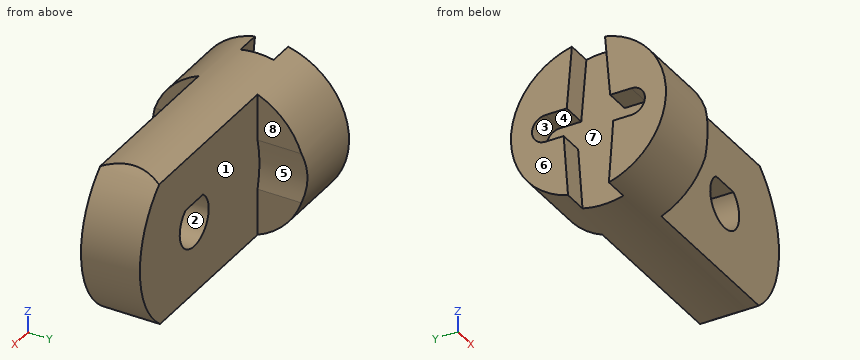
```python
from build123d import *

# Parameters (mm, degrees)
SKETCH_1_W                = 50
SKETCH_1_H                = 40
EXTRUDE_1_DEPTH           = 8
CHAMFER_1_SIZE            = 10
SKETCH_2_R                = 1.55
CUT_EXTRUDE_1_DEPTH       = 10
EXTRUDE_2_DEPTH           = 50
EXTRUDE_2_DEPTH_BACK      = 15
SKETCH_3_R                = 12.5
SKETCH_4_R                = 1.7
CUT_EXTRUDE_2_DEPTH       = 15
CUT_EXTRUDE_START         = -20
CUT_EXTRUDE_3_DEPTH       = 20
SKETCH_7_R                = 16.5
CUT_EXTRUDE_8_DEPTH       = 33
CUT_EXTRUDE_9_DEPTH       = 20
CHAMFER_3_SIZE            = 2
SKETCH_10_OUTSIDE_W       = 49.114
SKETCH_10_OUTSIDE_H       = 64.114
SKETCH_10_OUTSIDE_R       = 12.5
CUT_EXTRUDE_10_DEPTH      = 10
CHAMFER_4_SIZE            = 10
SKETCH_12_W               = 1.5
SKETCH_12_H               = 20
SKETCH_14_W               = 12
SKETCH_14_H               = 23
CUT_EXTRUDE_11_DEPTH      = 3
CUT_EXTRUDE_12_DEPTH      = 4.2
SKETCH_16_R               = 1.1
CUT_EXTRUDE_13_DEPTH      = 5
SKETCH_17_R               = 3.372674955
EXTRUDE_3_DEPTH           = 4
SKETCH_18_R               = 1.1
CUT_EXTRUDE_14_DEPTH      = 4
SKETCH_20_R               = 4
CUT_EXTRUDE_15_DEPTH      = 4
CUT_EXTRUDE_16_DEPTH      = 80.355214185
CUT_EXTRUDE_16_DEPTH_BACK = 80.355214185
SKETCH_21_W               = 47.755098741
SKETCH_21_H               = 76.122443719
SKETCH_26_R               = 4
CUT_EXTRUDE_19_DEPTH      = 20
SKETCH_28_W               = 34.99561618
SKETCH_28_H               = 41.128829021
CUT_EXTRUDE_20_DEPTH      = 10
SKETCH_29_W               = 7.599941767
SKETCH_29_H               = 6.479768366
EXTRUDE_6_DEPTH           = 9.5
SKETCH_24_R               = 12.607397707
CUT_EXTRUDE_21_DEPTH      = 15
CUT_EXTRUDE_22_DEPTH      = 4


# Read off the part's stored shape, not the designer's step: 切除-拉伸3
with BuildPart() as part:
    # 草图1 → 凸台-拉伸1 (new body)
    with BuildSketch(Plane.XY):
        Rectangle(SKETCH_1_W, SKETCH_1_H)
    extrude(amount=EXTRUDE_1_DEPTH)

    # 倒角1
    chamfer_1_edges = [part.edges().sort_by_distance(p)[0] for p in [
        (-25, -20, 4),
        (-25, 20, 4),
    ]]
    chamfer(chamfer_1_edges, length=CHAMFER_1_SIZE)

    # 草图2 → 切除-拉伸1 (cut)
    with BuildSketch(Plane.XY.offset(8)):
        with Locations((-2, -10)):
            Circle(SKETCH_2_R)
        with Locations((-2, 10)):
            Circle(SKETCH_2_R)
    extrude(amount=-CUT_EXTRUDE_1_DEPTH, mode=Mode.SUBTRACT)

    # 草图3 → 凸台-拉伸2 (add, two sides: drawn at the far end of the back side and taken through both)
    with BuildSketch(Plane(origin=(25, 0, 0), x_dir=(0, 0, -1), z_dir=(1, 0, 0)).offset(-EXTRUDE_2_DEPTH_BACK)):
        with Locations(Location((-4, 0, 0), (0, 0, 251.337075115))):
            Circle(SKETCH_3_R)
    extrude(amount=EXTRUDE_2_DEPTH + EXTRUDE_2_DEPTH_BACK)

    # 草图4 → 切除-拉伸2 (cut)
    with BuildSketch(Plane.XY.offset(8)):
        with Locations((-19.690178066, -4)):
            Circle(SKETCH_4_R)
        with Locations((-19.690178066, 4)):
            Circle(SKETCH_4_R)
    extrude(amount=-CUT_EXTRUDE_2_DEPTH, mode=Mode.SUBTRACT)

    # 切除-拉伸3 outline → 切除-拉伸3 (cut)
    with BuildSketch(Plane(origin=(75, 0, 0), x_dir=(0, 0, -1), z_dir=(1, 0, 0)).offset(CUT_EXTRUDE_START)):
        with BuildLine():
            Line((7.56233108, -4.75), (-15.56233108, -4.75))
            ThreePointArc((-15.56233108, -4.75), (-4, -12.5), (7.56233108, -4.75))
        make_face()
        with BuildLine():
            ThreePointArc((7.56233108, 4.75), (-4, 12.5), (-15.56233108, 4.75))
            Line((-15.56233108, 4.75), (7.56233108, 4.75))
        make_face()
    extrude(amount=CUT_EXTRUDE_3_DEPTH, mode=Mode.SUBTRACT)

    # 草图7 → 切除-拉伸8 (cut)
    with BuildSketch(Plane.XZ.offset(4.75)):
        with Locations((58.5, 4)):
            Circle(SKETCH_7_R)
    cut_extrude_8 = extrude(amount=CUT_EXTRUDE_8_DEPTH, mode=Mode.SUBTRACT)

    # 镜向1: 切除-拉伸8 across plane
    add(cut_extrude_8.mirror(Plane.ZX), mode=Mode.SUBTRACT)

    # 草图8 → 切除-拉伸9 (cut)
    with BuildSketch(Plane.XZ.offset(4.75)):
        with BuildLine():
            Line((60, 19.107397707), (75.764252489, 33.62580965))
            Line((75.764252489, 33.62580965), (78.826270749, -18.347337912))
            Line((78.826270749, -18.347337912), (60, -10.892602293))
            ThreePointArc((60, -10.892602293), (75, 4.107397707), (60, 19.107397707))
        make_face()
    extrude(amount=-CUT_EXTRUDE_9_DEPTH, mode=Mode.SUBTRACT)

    # 倒角3
    chamfer_3_edges = [part.edges().sort_by_distance(p)[0] for p in [
        (10, 0, 16.5),
        (10, 0, -8.5),
    ]]
    chamfer(chamfer_3_edges, length=CHAMFER_3_SIZE)

    # 草图10 outside → 切除-拉伸10 (cut)
    with BuildSketch(Plane(origin=(25, 0, 0), x_dir=(0, 0, -1), z_dir=(1, 0, 0))):
        with Locations((-4, 0)):
            Rectangle(SKETCH_10_OUTSIDE_W, SKETCH_10_OUTSIDE_H)
        with Locations((-4.107397707, 0)):
            Circle(SKETCH_10_OUTSIDE_R, mode=Mode.SUBTRACT)
    extrude(amount=-CUT_EXTRUDE_10_DEPTH, mode=Mode.SUBTRACT)

    # 倒角4
    # the kernel refuses this chamfer: 10 mm, written as the material it takes off along each edge
    with BuildSketch(Plane(origin=(15, -20, -25.71682988), x_dir=(-0.9996219169112968, -0.027495876610586317, 0), z_dir=(0, 0, 1))) as chamfer_4_piece_1_section:
        Polygon((CHAMFER_4_SIZE * 0.999621916911, -CHAMFER_4_SIZE * 0.0274958766106), (-CHAMFER_4_SIZE * 0.0274958766106, -CHAMFER_4_SIZE * 0.999621916911), (0, 0), align=None)
    chamfer_4_piece_1 = extrude(amount=59.433659759, mode=Mode.PRIVATE)
    chamfer_4_piece_1 = chamfer_4_piece_1 - Plane(origin=(11.669205873, 0, 4.107397707), x_dir=(0, 0, -1), z_dir=(1, 0, 0)) * Cylinder(12.5, 159, mode=Mode.PRIVATE)
    add(chamfer_4_piece_1, mode=Mode.SUBTRACT)
    with BuildSketch(Plane(origin=(15, 20, 33.71682988), x_dir=(-0.9996219169112968, 0.027495876610586317, 0), z_dir=(0, 0, -1))) as chamfer_4_piece_2_section:
        Polygon((CHAMFER_4_SIZE * 0.999621916911, -CHAMFER_4_SIZE * 0.0274958766106), (-CHAMFER_4_SIZE * 0.0274958766106, -CHAMFER_4_SIZE * 0.999621916911), (0, 0), align=None)
    chamfer_4_piece_2 = extrude(amount=59.433659759, mode=Mode.PRIVATE)
    chamfer_4_piece_2 = chamfer_4_piece_2 - Plane(origin=(11.669205873, 0, 4.107397707), x_dir=(0, 0, -1), z_dir=(1, 0, 0)) * Cylinder(12.5, 159, mode=Mode.PRIVATE)
    add(chamfer_4_piece_2, mode=Mode.SUBTRACT)

    # 草图12 → 切除-旋转2 (revolve, cut)
    with BuildSketch(Plane(origin=(0, 0, 0), x_dir=(1, 0, 0), z_dir=(0, 1, 0))):
        with Locations((14.75, 8.392602293)):
            Rectangle(SKETCH_12_W, SKETCH_12_H)
    revolve(axis=Axis((50, 0, 4.107397707), (-1, 0, 0)), mode=Mode.SUBTRACT)

    # 草图14 → 切除-拉伸11 (cut)
    with BuildSketch(Plane(origin=(0, 0, 0), x_dir=(-1, 0, 0), z_dir=(0, 0, -1))):
        with Locations((2, 4.65)):
            Rectangle(SKETCH_14_W, SKETCH_14_H)
    extrude(amount=-CUT_EXTRUDE_11_DEPTH, mode=Mode.SUBTRACT)

    # 草图15 → 切除-拉伸12 (cut)
    with BuildSketch(Plane(origin=(0, 0, 3), x_dir=(-1, 0, 0), z_dir=(0, 0, -1))):
        with BuildLine():
            ThreePointArc((4.631967524, 4.49702381), (2, 16.1), (-0.631967524, 4.49702381))
            ThreePointArc((-0.631967524, 4.49702381), (2, 0.95), (4.631967524, 4.49702381))
        make_face()
    extrude(amount=-CUT_EXTRUDE_12_DEPTH, mode=Mode.SUBTRACT)

    # 草图16 → 切除-拉伸13 (cut)
    with BuildSketch(Plane(origin=(0, 0, 0), x_dir=(-1, 0, 0), z_dir=(0, 0, -1))):
        with Locations((2, 18.3)):
            Circle(SKETCH_16_R)
    extrude(amount=-CUT_EXTRUDE_13_DEPTH, mode=Mode.SUBTRACT)

    # 草图17 → 凸台-拉伸3 (add)
    with BuildSketch(Plane(origin=(0, 0, 0), x_dir=(-1, 0, 0), z_dir=(0, 0, -1))):
        with Locations((2, -10)):
            Circle(SKETCH_17_R)
    extrude(amount=-EXTRUDE_3_DEPTH)

    # 草图18 → 切除-拉伸14 (cut)
    with BuildSketch(Plane(origin=(0, 0, 0), x_dir=(-1, 0, 0), z_dir=(0, 0, -1))):
        with Locations((2, -9)):
            Circle(SKETCH_18_R)
    extrude(amount=-CUT_EXTRUDE_14_DEPTH, mode=Mode.SUBTRACT)

    # 草图20 → 切除-拉伸15 (cut)
    with BuildSketch(Plane(origin=(0, 0, 7.2), x_dir=(-1, 0, 0), z_dir=(0, 0, -1))):
        with Locations((2, 10)):
            Circle(SKETCH_20_R)
    extrude(amount=-CUT_EXTRUDE_15_DEPTH, mode=Mode.SUBTRACT)

    # 草图21 → 切除-拉伸16 (cut, two sides: drawn at the far end of the back side and taken through both)
    with BuildSketch(Plane(origin=(0, 0, 0), x_dir=(-1, 0, 0), z_dir=(0, 0, -1)).offset(-CUT_EXTRUDE_16_DEPTH_BACK)):
        with Locations((8.377549371, -2.117346793)):
            Rectangle(SKETCH_21_W, SKETCH_21_H)
    extrude(amount=CUT_EXTRUDE_16_DEPTH + CUT_EXTRUDE_16_DEPTH_BACK, mode=Mode.SUBTRACT)

    # 草图26 → 切除-拉伸19 (cut)
    with BuildSketch(Plane.XZ.offset(4.75)):
        with Locations((60, 4.107397707)):
            Circle(SKETCH_26_R)
    extrude(amount=-CUT_EXTRUDE_19_DEPTH, mode=Mode.SUBTRACT)

    # 草图28 → 切除-拉伸20 (cut)
    with BuildSketch(Plane.XZ.offset(4.75)):
        with Locations((60, 4.107397707)):
            Rectangle(SKETCH_28_W, SKETCH_28_H)
    cut_extrude_20 = extrude(amount=CUT_EXTRUDE_20_DEPTH, mode=Mode.SUBTRACT)

    # 镜向2: 切除-拉伸20 across plane
    add(cut_extrude_20.mirror(Plane.ZX), mode=Mode.SUBTRACT)

    # 草图29 → 凸台-拉伸6 (add)
    with BuildSketch(Plane.XZ.offset(4.75)):
        with Locations((61.399970884, 10.54728189)):
            Rectangle(SKETCH_29_W, SKETCH_29_H)
    extrude(amount=-EXTRUDE_6_DEPTH)

    # 草图24 → 切除-拉伸21 (cut)
    with BuildSketch(Plane.ZY.offset(-15.5)):
        with Locations((4.107397707, 0)):
            Circle(SKETCH_24_R)
    extrude(amount=-CUT_EXTRUDE_21_DEPTH, mode=Mode.SUBTRACT)

    # 草图30 → 切除-拉伸22 (cut)
    with BuildSketch(Plane.ZY.offset(-30.5)):
        with BuildLine():
            Line((6.307397707, -6.9), (6.307397707, 6.9))
            ThreePointArc((6.307397707, 6.9), (4.107397707, 9.1), (1.907397707, 6.9))
            Line((1.907397707, 6.9), (1.907397707, -6.9))
            ThreePointArc((1.907397707, -6.9), (4.107397707, -9.1), (6.307397707, -6.9))
        make_face()
        with BuildLine():
            Line((-8.058924565, -3.29125179), (1.907397707, -4))
            Line((1.907397707, -4), (1.907397707, 4))
            Line((1.907397707, 4), (-8.058924565, 3.29125179))
            ThreePointArc((-8.058924565, 3.29125179), (-8.5, 0), (-8.058924565, -3.29125179))
        make_face()
        with BuildLine():
            Line((6.307397707, 3.5), (6.307397707, -3.5))
            Line((6.307397707, -3.5), (16.211202868, -2.671427431))
            ThreePointArc((16.211202868, -2.671427431), (16.427590994, -1.343496214), (16.5, 0))
            ThreePointArc((16.5, 0), (16.427590994, 1.343496214), (16.211202868, 2.671427431))
            Line((16.211202868, 2.671427431), (6.307397707, 3.5))
        make_face()
    extrude(amount=-CUT_EXTRUDE_22_DEPTH, mode=Mode.SUBTRACT)


solid = part.part
```
Work out the finished part from the listing and answer in its coordinate system (mm). Face numbers are marked on the shaded views. A direction names the side the tool comes from. Round coordinates to 2 decimals unless told otherwise and drop trailing zeros. Write each loop counter-clockwise with the first axis right and the second up, starting at its lowest first coordinate (ties: lowest second). Pieces come first, ordered by that corner, then holes. Notation, with made-up numbers: (33.25, 48) -> (67.25, 48) arc R24 cw to (67.25, 63) -> close; hole circle Ø9 at (-2, 31). An arc over 180 degrees is marked (long way). Write each question's results on one line, items separated by ' | '.
Q1. Flat-ended cylindrical pins translate along their axes: P1, Ø11.5, axis at x = 53.5, z = 0, coming from the +Y side; P2, Ø8, axis at x = 60, y = -8, coming from the -Z side; P3, Ø2, axis at x = 41.5, y = -8.5, coming from the -Z side; P4, Ø12, axis at y = 1, z = 13, coming from the -X side. Find the tip coordinate at first contact, or state that the pin passes through.
Data:
P1: y = 4.75 | P2: z = -7.84 | P3: z = -6 | P4: x = 30.5
Q2. Section B-B, the plane z = 4.75 is taken. Write down the section's boundary in (x, y), then the cut area to 3 significant figures.
Data:
outline: (30.5, -12.48) -> (42.02, -12.48) -> (42.02, -4.75) -> (56.05, -4.75) -> (56.05, 4.75) -> (42.02, 4.75) -> (42.02, 12.48) -> (30.5, 12.48) -> (30.5, 9) -> (34.5, 9) -> (34.5, -9) -> (30.5, -9) -> close; (63.95, -4.75) -> (74.99, -4.75) -> (74.99, 4.75) -> (63.95, 4.75) -> close | area: 454 mm^2
Q3. Straight lines are drawn through the part: line 1 along Y through (x, z) = (51.5, -3.25); line 2 along Z through (x, y) = (60, 0.25); line 3 along Y through (x, z) = (33, -3.5). For each, find the intervals that lie inside material, in ascending order. Write a range as [from, to].
Data:
line 1: [-4.75, 4.75] | line 2: [-8.5, 0.11], [7.31, 16.5] | line 3: [-10, -3.62], [3.62, 10]
Q4. Section D-D, the plane y = 2 is taken. Write down the section's boundary in (x, z), then the cut area to 3 significant figures.
Data:
outline: (34.5, -8.34) -> (68.37, -8.34) arc R15 ccw to (68.68, 16.34) -> (34.5, 16.34) -> close; hole (57.6, 7.31) arc R4 ccw (long way) to (62.4, 7.31) -> close | area: 904 mm^2
Q5. Section C-C, the plane y = -7.5 is taken. Write down the section's boundary in (x, z).
Data:
outline: (30.5, -6) -> (42.5, -6) -> (42.5, -0.04) arc R16.5 cw to (42.5, 8.04) -> (42.5, 14) -> (30.5, 14) -> (30.5, 6.22) -> (34.5, 6.22) -> (34.5, 1.99) -> (30.5, 1.99) -> close
Q6. Which of the six approach directions +Z, -Z, +X, -X, +Y, -Y give full straight-line access (tool end or side, diameter ignored) to the marked faces 5, 6, 7 and 8?
Data:
face 5: +X, +Y | face 6: +Z, -Z, -X, +Y, -Y | face 7: -X | face 8: +Z, -Z, +X, +Y
Q7. Determine the mould class of the marked faces 1, 2, 3 and 4 for opening direction Y: released by +Y, released by -Y, zero draft, split by the parting line, or undercut.
Data:
face 1: released by +Y | face 2: zero draft | face 3: undercut | face 4: undercut
Q8. Section A-A, the plane x = 60 is taken. Write down the section's boundary in (y, z).
Data:
outline: (-4.75, -7.56) arc R12.5 ccw to (4.75, -7.56) -> (4.75, 0.11) -> (-4.75, 0.11) -> close; (-4.75, 7.31) -> (4.75, 7.31) -> (4.75, 15.56) arc R12.5 ccw to (-4.75, 15.56) -> close
